Check sheet for the modelled part. Datum: model origin and axes. Units: mm. Round coordinates to 2 decimals unless told otherwise and drop trailing zeros. Loops run counter-clockwise (first coordinate to the right, second up) from the corner with the lowest first, then second, coordinate; pieces in that order, holes last. Notation, with made-up numbers: (68, 12.5) - (125, 12.5) arc R27 ccw to (125, 36.5) - close; hole circle Ø4 at (8.25, -29.75). An arc over 180 degrees is marked (long way). Put each result on its own line as item: value. Start each with the question number.
Item 1: Section check A-A, the plane z = 0. Record the cut outline in (x, y).
Item 2: Gauge pin test, flat ends, axial feed: pin 1 Ø1.5 at (x, z) = (74, -1) entering from +Y; pin 2 Ø4 at (y, z) = (-5, -3.5) entering from +X; pin 3 Ø2.5 at (x, z) = (-73, 1) entering from -Y. Record the tip position at first contact, or that the pin passes through.
Item 3: Material ranges on line 1 along X through (y, z) = (6.5, 4.5); line 2 along X through (y, z) = (-2.75, 3.25); line 3 along Y through (x, z) = (45, -2), recorded low to high.
Item 4: Section check B-B, the plane x = -26. Record the cut outline in (y, z), and give its area (3 significant figures).
from build123d import *

# Parameters (mm, degrees)
F0_R      = 4
F1_DEPTH  = 69.977
F2_R      = 8
F3_DEPTH  = 1
F5_DEPTH  = 5
F6_R      = 4
F7_DEPTH  = 5
F8_R      = 8
F9_DEPTH  = 1
F11_DEPTH = 5
F12_R     = 4
F13_DEPTH = 5


with BuildPart() as f1:
    # F0 (on Right) → F1 (new body, symmetric)
    with BuildSketch(Plane.YZ):
        Circle(F0_R)
    extrude(amount=F1_DEPTH, both=True)

    # F2 (on face) → F3 (join)
    with BuildSketch(Plane.YZ.offset(69.977)):
        Circle(F2_R)
    extrude(amount=F3_DEPTH)

    # F4 (on face) → F5 (join)
    with BuildSketch(Plane.YZ.offset(70.977)):
        Polygon((6, 3.4641016151), (0, 6.9282032303), (-6, 3.4641016151), (-6, -3.4641016151), (0, -6.9282032303), (6, -3.4641016151), align=None)
    extrude(amount=F5_DEPTH)

    # F6 (on face) → F7 (join)
    with BuildSketch(Plane.YZ.offset(75.977)):
        Circle(F6_R)
    extrude(amount=F7_DEPTH)

    # F8 (on face) → F9 (join)
    with BuildSketch(Plane(origin=(-69.977, 0, 0), x_dir=(0, -1, 0), z_dir=(-1, 0, 0))):
        Circle(F8_R)
    extrude(amount=F9_DEPTH)

    # F10 (on face) → F11 (join)
    with BuildSketch(Plane(origin=(-70.977, 0, 0), x_dir=(0, -1, 0), z_dir=(-1, 0, 0))):
        Polygon((0, -6.9282032303), (6, -3.4641016151), (6, 3.4641016151), (0, 6.9282032303), (-6, 3.4641016151), (-6, -3.4641016151), align=None)
    extrude(amount=F11_DEPTH)

    # F12 (on face) → F13 (join)
    with BuildSketch(Plane(origin=(-75.977, 0, 0), x_dir=(0, -1, 0), z_dir=(-1, 0, 0))):
        Circle(F12_R)
    extrude(amount=F13_DEPTH)


solid = f1.part
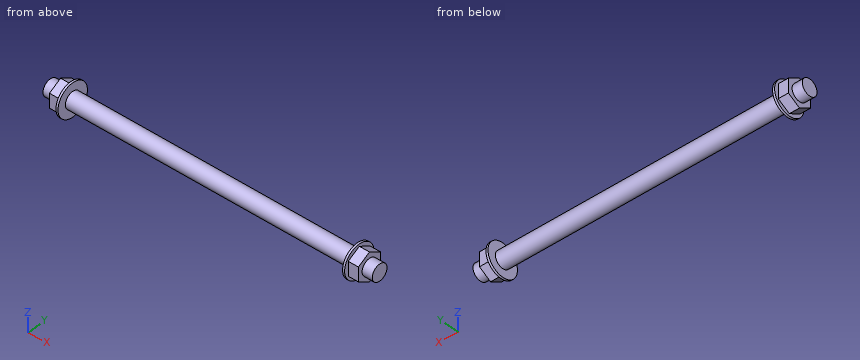
Check result:
1. outline: (-80.98, -4) - (-75.98, -4) - (-75.98, -6) - (-70.98, -6) - (-70.98, -8) - (-69.98, -8) - (-69.98, -4) - (69.98, -4) - (69.98, -8) - (70.98, -8) - (70.98, -6) - (75.98, -6) - (75.98, -4) - (80.98, -4) - (80.98, 4) - (75.98, 4) - (75.98, 6) - (70.98, 6) - (70.98, 8) - (69.98, 8) - (69.98, 4) - (-69.98, 4) - (-69.98, 8) - (-70.98, 8) - (-70.98, 6) - (-75.98, 6) - (-75.98, 4) - (-80.98, 4) - close
2. pin 1: y = 6
2. pin 2: x = 75.98
2. pin 3: y = -6
3. line 1: -70.98 to -69.98, 69.98 to 70.98
3. line 2: -75.98 to -69.98, 69.98 to 75.98
3. line 3: -3.46 to 3.46
4. outline: circle Ø8 at (0, 0)
4. area: 50.3 mm²
